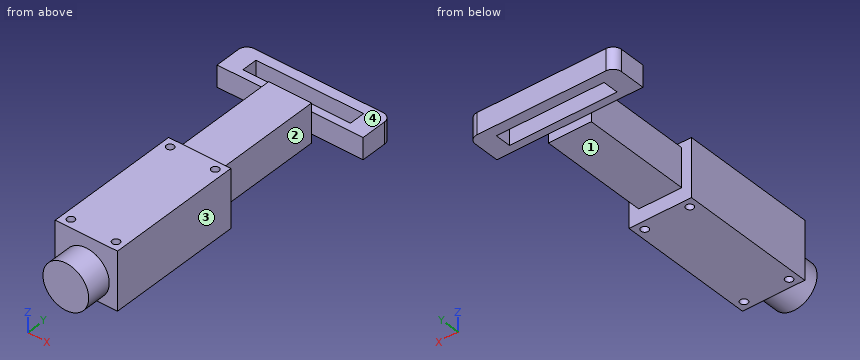
```python
from build123d import *

# Parameters (mm, degrees)
SKETCH_1_W                  = 29
SKETCH_1_H                  = 64
EXTRUDE_1_DEPTH             = 27
SKETCH_2_W                  = 20
SKETCH_2_H                  = 18
EXTRUDE_2_DEPTH             = 51
SKETCH_3_W                  = 44
SKETCH_3_H                  = 10
EXTRUDE_3_DEPTH             = 16
SKETCH_4_W                  = 10
SKETCH_4_H                  = 16
EXTRUDE_4_DEPTH             = 24
SKETCH_5_W                  = 50.1
SKETCH_5_H                  = 7.4
CUT_EXTRUDE_1_DEPTH         = 21.6
SKETCH_6_W                  = 10.65
SKETCH_6_H                  = 11.6
HOLE_WIZARD_3_5_3_5_1_D     = 3.5
HOLE_WIZARD_3_5_3_5_1_DEPTH = 27
FILLET_1_R                  = 4


with BuildPart() as part:
    # 草图1 → 凸台-拉伸1 (new body)
    with BuildSketch(Plane.XY.offset(13.5)):
        Rectangle(SKETCH_1_W, SKETCH_1_H)
    extrude(amount=-EXTRUDE_1_DEPTH)

    # 草图2 → 凸台-拉伸2 (add)
    with BuildSketch(Plane(origin=(0, 32, 0), x_dir=(-1, 0, 0), z_dir=(0, 1, 0))):
        with Locations((0, 2.1)):
            Rectangle(SKETCH_2_W, SKETCH_2_H)
    extrude(amount=EXTRUDE_2_DEPTH)

    # 草图3 → 凸台-拉伸3 (add)
    with BuildSketch(Plane(origin=(0, 83, 0), x_dir=(-1, 0, 0), z_dir=(0, 1, 0))):
        with Locations((12, 2.1)):
            Rectangle(SKETCH_3_W, SKETCH_3_H)
    extrude(amount=EXTRUDE_3_DEPTH)

    # 草图4 → 凸台-拉伸4 (add)
    with BuildSketch(Plane(origin=(10, 0, 0), x_dir=(0, 0, -1), z_dir=(1, 0, 0))):
        with Locations((-2.1, 91)):
            Rectangle(SKETCH_4_W, SKETCH_4_H)
    extrude(amount=EXTRUDE_4_DEPTH)

    # 草图5 → 切除-拉伸1 (cut, through all)
    with BuildSketch(Plane.XY.offset(7.1)):
        with Locations((0, 90.4)):
            Rectangle(SKETCH_5_W, SKETCH_5_H)
    extrude(amount=-CUT_EXTRUDE_1_DEPTH, mode=Mode.SUBTRACT)

    # 草图6 → 旋转1 (revolve)
    with BuildSketch(Plane.XY.offset(-2.7)):
        with Locations((5.325, -37.8)):
            Rectangle(SKETCH_6_W, SKETCH_6_H)
    revolve(axis=Axis((0, -32, -2.7), (0, -1, 0)))

    # Ø3.5 (3.5) 直径孔1
    with Locations(Plane.XY.offset(13.5)):
        with Locations((-10.5, -28), (10.5, -28), (-10.5, 28), (10.5, 28)):
            Hole(HOLE_WIZARD_3_5_3_5_1_D / 2, depth=HOLE_WIZARD_3_5_3_5_1_DEPTH)

    # 圆角1
    fillet_1_edges = [part.edges().sort_by_distance(p)[0] for p in [
        (-34, 99, 2.1),
        (34, 99, 2.1),
    ]]
    fillet(fillet_1_edges, radius=FILLET_1_R)


solid = part.part
```
Build history of the part. All positions in model axes, mm. Face numbers are marked on the shaded views. A direction names the side the tool comes from. Give positions to 0.01 mm unless a question says otherwise; leave off trailing zeros. Loops run counter-clockwise (first coordinate to the right, second up) from the corner with the lowest first, then second, coordinate; pieces in that order, holes last.
1) Band-saw the part on C-C on z = -10.75. List the corners of the cut face in (x, y), then the cut area to 3 significant figures.
Values follow:
outline: (-14.5, -32) - (-6.97, -32) - (-6.97, -43.6) - (6.97, -43.6) - (6.97, -32) - (14.5, -32) - (14.5, 32) - (-14.5, 32) - close; hole circle Ø3.5 at (-10.5, -28); hole circle Ø3.5 at (-10.5, 28); hole circle Ø3.5 at (10.5, -28); hole circle Ø3.5 at (10.5, 28)
area: 1,980 mm2
2) Band-saw the part on A-A on y = 28. List the corners of the cut face in (x, z), then the cut area to 3 significant figures.
Values follow:
outline: (-14.5, -13.5) - (-12.25, -13.5) - (-12.25, 13.5) - (-14.5, 13.5) - close; (-8.75, -13.5) - (8.75, -13.5) - (8.75, 13.5) - (-8.75, 13.5) - close; (12.25, -13.5) - (14.5, -13.5) - (14.5, 13.5) - (12.25, 13.5) - close
area: 594 mm2
3) Band-saw the part on B-B on x = 0. List the corners of the cut face in (y, z).
Values follow:
outline: (-43.6, -13.35) - (-32, -13.35) - (-32, -13.5) - (32, -13.5) - (32, -6.9) - (83, -6.9) - (83, -2.9) - (86.7, -2.9) - (86.7, 7.1) - (83, 7.1) - (83, 11.1) - (32, 11.1) - (32, 13.5) - (-32, 13.5) - (-32, 7.95) - (-43.6, 7.95) - close; (94.1, -2.9) - (99, -2.9) - (99, 7.1) - (94.1, 7.1) - close
4) Band-saw the part on D-D on z = 5. List the corners of the cut face in (x, y), then the cut area to 3 significant figures.
Values follow:
outline: (-34, 83) - (-10, 83) - (-10, 32) - (-14.5, 32) - (-14.5, -32) - (-7.36, -32) - (-7.36, -43.6) - (7.36, -43.6) - (7.36, -32) - (14.5, -32) - (14.5, 32) - (10, 32) - (10, 83) - (34, 83) - (34, 95) arc R4 ccw to (30, 99) - (-30, 99) arc R4 ccw to (-34, 95) - close; hole (-25.05, 86.7) - (25.05, 86.7) - (25.05, 94.1) - (-25.05, 94.1) - close; hole circle Ø3.5 at (-10.5, -28); hole circle Ø3.5 at (-10.5, 28); hole circle Ø3.5 at (10.5, -28); hole circle Ø3.5 at (10.5, 28)
area: 3,720 mm2
5) Drop flat-ended pins along their axis: P1, Ø8, axis at x = -22, z = 4, coming from the -Y side; P2, Ø17.5, axis at x = -2.5, y = 89, coming from the -Z side; P3, Ø1, axis at y = -14, z = -2, coming from the -X side; P4, Ø3, axis at x = -10.5, y = -28, coming from the +Z side. Give the stop position or say it passes through.
Values follow:
P1: stops at y = 83
P2: stops at z = -6.9
P3: stops at x = -14.5
P4: passes through
6) 3-axis set-ups, long thin cutter, end or side, ignore diameter. For the marked faces 1, 2, 3 and 4: which of +Z, -Z, +X, -X, +Y, -Y reach the whole face in a straight line?
Values follow:
face 1: -Z, +X, -X, +Y
face 2: +Z, -Z, +X
face 3: +Z, -Z, +X, -Y
face 4: +Z, +X, -X, +Y
7) Probe line 1 along Y through (x, z) = (-10.5, 5.75); line 2 along Y through (x, z) = (10.5, -6.5); line 3 along Y through (x, z) = (-8, 11). List the from-to ranges inside material, lowest first.
Values follow:
line 1: y = -32 to -29.75, -26.25 to 26.25, 29.75 to 32, 83 to 86.7, 94.1 to 99
line 2: y = -32 to -29.75, -26.25 to 26.25, 29.75 to 32
line 3: y = -32 to 83
